Could you check a few things on this drawing? It's one solid part, dimensions in mm from its lowest x, y, z. A direction names the side the tool comes from. Coordinates: 2 decimals unless noted, no trailing zeros. Order: outer loops, then holes, each group sorted by start corner. A loop starts at its lowest first (then second) coordinate and runs counter-clockwise, first axis right, second up. Notation, with made-up numbers: (-39.75, -34.75) -> (14.25, -34.75) arc R20 ccw to (14.25, -17.75) -> close; hole circle Ø3 at (47.5, 42.25). An arc over 180 degrees is marked (long way). Answer as CSV lines item,"result".
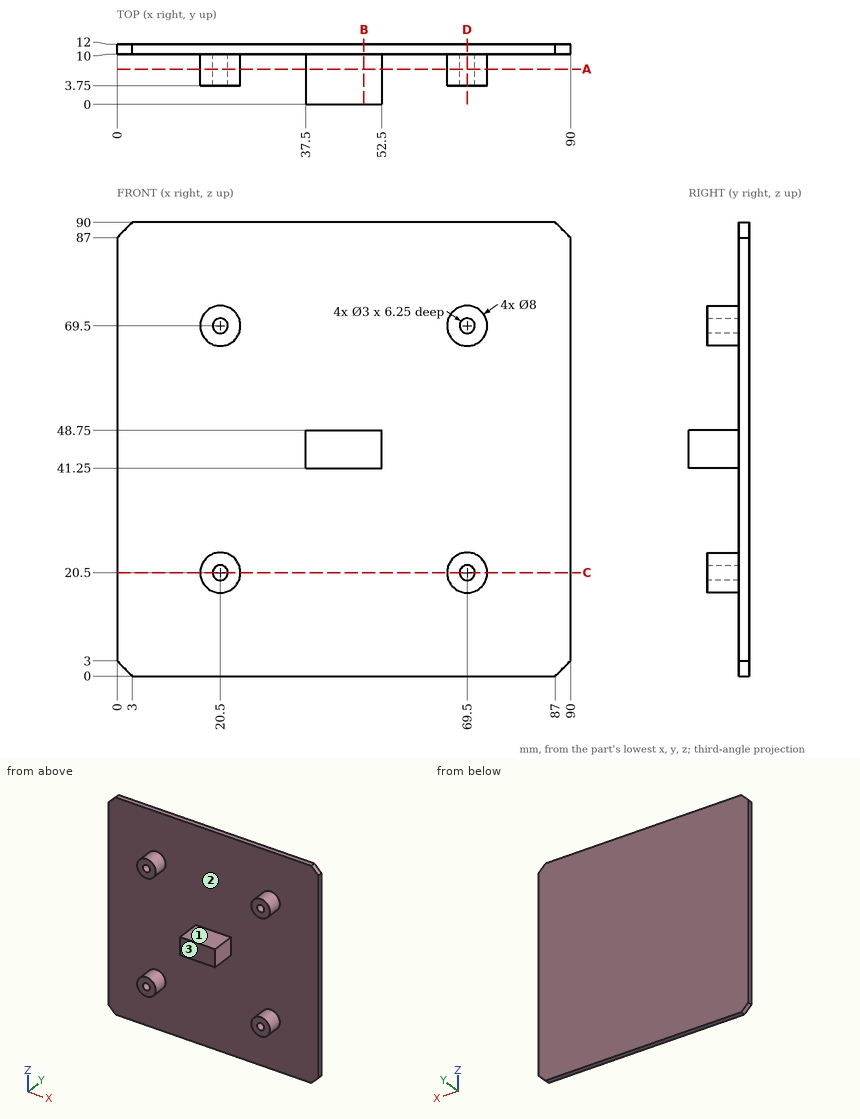
Q1. Imagine slicing it at A-A (y = 7). Give the number of separate pieces and of enclosed holes in the cut face, and give its area (3 significant figures).
Solution:
separate pieces,"5"
enclosed holes,"4"
area,"285 mm2"
Q2. Imagine slicing it at D-D (x = 69.5). List the corners of the cut face in (y, z) for me, and give its area (4 significant figures).
Solution:
outline,"(3.75, 16.5) -> (10, 16.5) -> (10, 0) -> (12, 0) -> (12, 90) -> (10, 90) -> (10, 73.5) -> (3.75, 73.5) -> (3.75, 71) -> (10, 71) -> (10, 68) -> (3.75, 68) -> (3.75, 65.5) -> (10, 65.5) -> (10, 24.5) -> (3.75, 24.5) -> (3.75, 22) -> (10, 22) -> (10, 19) -> (3.75, 19) -> close"
area,"242.5 mm2"
Q3. For P1, Ø1.5, axis at x = 69, z = 20.5, coming from the -Y side; P2, Ø2.5, axis at x = 71, z = 21.5, coming from the -Y side; P3, Ø10, axis at x = 44, z = 53, coming from the -Y side; P4, Ø6, axis at y = 4.5, z = 44, coming from the +X side, each with a flat end and sliding along its axis, tell me the tip position at first contact or that it passes through.
Solution:
P1,"y = 10"
P2,"y = 3.75"
P3,"y = 0"
P4,"x = 52.5"
Q4. Which directions (+Z, -Z, +X, -X, +Y, -Y) give clear straight access to the entire face, cutting with the end or side of a thin tool? Please do the marked faces 1, 2 and 3.
Solution:
face 1,"+Z, +X, -X, -Y"
face 2,"-Y"
face 3,"+Z, -Z, +X, -X, -Y"
Q5. If I drill on line 1 (X direction, y = 5, z = 20.5); line 2 (Y direction, x = 85.5, z = 78); line 3 (X direction, y = 8.5, z = 17), over which ranges is the centre line in solid material (lowest first)?
Solution:
line 1,"16.5 to 19, 22 to 24.5, 65.5 to 68, 71 to 73.5"
line 2,"10 to 12"
line 3,"18.56 to 22.44, 67.56 to 71.44"
Q6. Imagine slicing it at B-B (x = 49). List the corners of the cut face in (y, z) for me, and give its area (3 significant figures).
Solution:
outline,"(0, 41.25) -> (10, 41.25) -> (10, 0) -> (12, 0) -> (12, 90) -> (10, 90) -> (10, 48.75) -> (0, 48.75) -> close"
area,"255 mm2"
Q7. Imagine slicing it at C-C (z = 20.5). List the corners of the cut face in (x, y) for me, and give its area (4 significant figures).
Solution:
outline,"(0, 10) -> (16.5, 10) -> (16.5, 3.75) -> (19, 3.75) -> (19, 10) -> (22, 10) -> (22, 3.75) -> (24.5, 3.75) -> (24.5, 10) -> (65.5, 10) -> (65.5, 3.75) -> (68, 3.75) -> (68, 10) -> (71, 10) -> (71, 3.75) -> (73.5, 3.75) -> (73.5, 10) -> (90, 10) -> (90, 12) -> (0, 12) -> close"
area,"242.5 mm2"
